Autodesk Inventor part; units mm, degrees
ref_plane "YZ Plane" through (0, 0, 0) normal (1, 0, 0) x (0, 1, 0)
ref_plane "XZ Plane" through (0, 0, 0) normal (0, 1, 0) x (-1, 0, 0)
ref_plane "XY Plane" through (0, 0, 0) normal (0, 0, 1) x (1, 0, 0)
sketch "Sketch1" plane through (0, 0, 0) normal (0, 0, 1) x (1, 0, 0)
  line L0 (-27, -64) -> (27, -64)
  line L1 (27, -64) -> (27, 64)
  line L2 (27, 64) -> (-27, 64)
  line L3 (-27, 64) -> (-27, -64)
  line L4 (-27, -64) -> (27, 64) construction
  line L5 (27, -64) -> (-27, 64) construction
  line L6 (-13, 56) -> (13, 56)
  line L7 (19, 50) -> (19, 41)
  line L8 (13, 35) -> (13, 35)
  line L9 (-19, 41) -> (-19, 50)
  arc A0 (-13, 56) -> (-19, 50) centre (-13, 50) ccw
  arc A1 (19, 50) -> (13, 56) centre (13, 50) ccw
  arc A2 (13, 35) -> (19, 41) centre (13, 41) ccw
  arc A3 (-19, 41) -> (-13, 35) centre (-13, 41) ccw
  line L10 (-37.8, 0) -> (37.8, 0) construction
  line L11 (-27, 64) -> (27, -64) construction
  line L12 (-13, -56) -> (13, -56)
  line L13 (19, -50) -> (19, -41)
  line L14 (13, -35) -> (13, -35)
  line L15 (-19, -41) -> (-19, -50)
  arc A4 (-19, -50) -> (-13, -56) centre (-13, -50) ccw
  arc A5 (13, -56) -> (19, -50) centre (13, -50) ccw
  arc A6 (19, -41) -> (13, -35) centre (13, -41) ccw
  arc A7 (-13, -35) -> (-19, -41) centre (-13, -41) ccw
  line L16 (-13, 35) -> (-13, -35)
  line L17 (13, 35) -> (13, -35)
  line L18 (0, -89.6) -> (0, 89.6) construction
  line L19 (-13, 35) -> (-13, 35)
  line L20 (13, 35) -> (-13, 35) construction
  line L21 (-13, -35) -> (-13, -35)
  line L22 (13, -35) -> (-13, -35) construction
  point P0 (0, 0)
  point P1 (0, 56)
  point P2 (0, 0)
  point P3 (13, 35)
  point P4 (13, -35)
  point P5 (-13, -35)
  point P6 (-13, 35)
  dimension "d0" = 54
  dimension "d1" = 128
  dimension "d2" = 38
  dimension "d3" = 6
  dimension "d4" = 35
  dimension "d5" = 8
  dimension "d6" = 26
extrude "Extrusion1" add sketch "Sketch1" along normal mid plane 40
fillet "Fillet1" radius 14 4 edges at (27, -64, 0) (-27, -64, 0) (-27, 64, 0) (27, 64, 0)
sketch "Sketch2" plane through (27, -50, 20) normal (1, 0, 0) x (0, 0, -1)
  line L0 (0, 0) -> (0, 100)
  line L1 (40, 100) -> (40, 0)
  arc A0 (0, 35) -> (4.6393, 30.2757) centre (20, 50) ccw
  arc A1 (0, 65) -> (0, 35) centre (20, 50) ccw construction
  arc A2 (40, 65) -> (35.3607, 69.7243) centre (20, 50) ccw
  arc A3 (40, 35) -> (40, 65) centre (20, 50) ccw construction
  line L2 (0, 65) -> (0, 35)
  line L3 (0, 15) -> (0, 85)
  line L4 (40, 85) -> (40, 15)
  line L5 (40, 65) -> (40, 35)
  circle A4 centre (20, 50) radius 18 construction
  line L6 (11.1075, 74.432) -> (20, 50) construction
  line L7 (28.8925, 74.432) -> (20, 50) construction
  line L8 (20, -39.6) -> (20, 139.6) construction
  line L9 (11.1075, 74.432) -> (28.8925, 74.432) construction
  arc A5 (26.1564, 66.9145) -> (13.8436, 66.9145) centre (20, 50) ccw
  arc A6 (4.6393, 69.7243) -> (13.8436, 66.9145) centre (11.1075, 74.432) ccw
  arc A7 (19.1075, 74.432) -> (19.0885, 74.9834) centre (11.1075, 74.432) ccw construction
  arc A8 (20.9115, 74.9834) -> (20.8925, 74.432) centre (28.8925, 74.432) ccw construction
  arc A9 (26.1564, 66.9145) -> (35.3607, 69.7243) centre (28.8925, 74.432) ccw
  arc A10 (4.6393, 69.7243) -> (0, 65) centre (20, 50) ccw
  arc A11 (35.3607, 69.7243) -> (4.6393, 69.7243) centre (20, 50) ccw construction
  line L10 (55, 50) -> (-15, 50) construction
  circle A12 centre (20, 50) radius 18 construction
  line L11 (11.1075, 25.568) -> (20, 50) construction
  line L12 (28.8925, 25.568) -> (20, 50) construction
  line L13 (20, 139.6) -> (20, -39.6) construction
  arc A13 (13.8436, 33.0855) -> (26.1564, 33.0855) centre (20, 50) ccw
  arc A14 (13.8436, 33.0855) -> (4.6393, 30.2757) centre (11.1075, 25.568) ccw
  arc A15 (35.3607, 30.2757) -> (26.1564, 33.0855) centre (28.8925, 25.568) ccw
  arc A16 (4.6393, 30.2757) -> (35.3607, 30.2757) centre (20, 50) ccw construction
  arc A17 (35.3607, 30.2757) -> (40, 35) centre (20, 50) ccw
  point P0 (20, 74.432)
  dimension "d10" = 50
  dimension "d11" = 36
  dimension "d15" = 40
extrude "Extrusion2" add sketch "Sketch2" along normal blind 12
sketch "Sketch3" plane through (39, -50, 20) normal (1, 0, 0) x (0, 0, -1)
  arc A0 (40, 65) -> (35.3607, 69.7243) centre (20, 50) ccw
  circle A1 centre (20, 50) radius 15
  dimension "d18" = 30
extrude "Extrusion3" add sketch "Sketch3" along normal blind 25
chamfer "Chamfer1" distance 2 angle 45 1 edges at (64, 0, 15)
mirror "Mirror1" about plane through (0, 0, 0) normal (1, 0, 0) of "Extrusion2", "Extrusion3", "Chamfer1"
sketch "Sketch4" plane through (-64, 0, 0) normal (-1, 0, 0) x (0, 0, 1)
  circle A0 centre (0, 0) radius 13
  point P0 (0, 0)
hole "Hole1" at (-64, 0, 0) direction (1, 0, 0) diameter 15 end through all
properties part number "Part036.Connecting cross" material "Steel, Carbon"
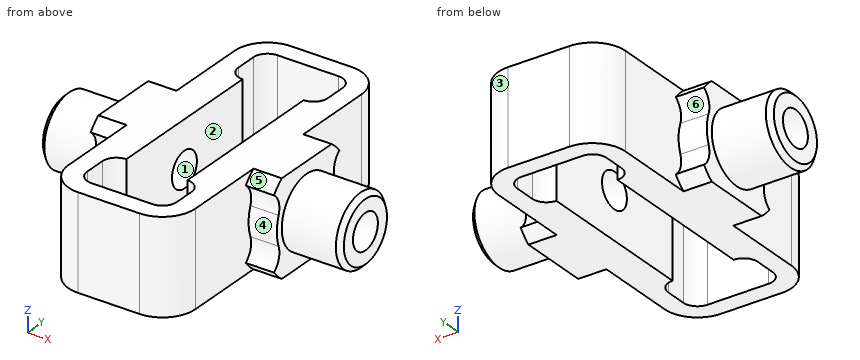
Input: part model. Units: mm. Frame: model coordinates. Face numbers are marked on the shaded views. A direction names the side the tool comes from. Give positions to 0.01 mm unless a question says otherwise; leave off trailing zeros. Order: outer loops, then holes, each group sorted by start corner. A loop starts at its lowest first (then second) coordinate and runs counter-clockwise, first axis right, second up. Notation, with made-up numbers: (67.5, -33.5) - (95.5, -33.5) arc R11 ccw to (95.5, -20.5) - close; hole circle Ø6 at (69.25, 37.25). An arc over 180 degrees is marked (long way). One line per item, written item: value.
1. Draft query along X for the marked faces 1, 2 and 3. Return one class per face: released by +X, released by -X, zero draft, split by the parting line, or undercut.
Determined:
face 1: zero draft
face 2: undercut
face 3: released by +X
2. Reachability of the marked faces 4, 5 and 6 from +Z, -Z, +X, -X, +Y, -Y: full face, straight path, thin tool, end or side. Return the list, or none.
Determined:
face 4: +X, -Y
face 5: +Z, +X, -Y
face 6: -X, +Y
3. Cut plane D-D, the plane x = -30.5. Output: boundary loops of the cut face in (y, z), and give its area (3 significant figures).
Determined:
outline: (-19.72, -15.36) arc R25 ccw to (-15, -20) - (15, -20) arc R25 ccw to (19.72, -15.36) arc R8 cw to (16.91, -6.16) arc R18 ccw to (16.91, 6.16) arc R8 cw to (19.72, 15.36) arc R25 ccw to (15, 20) - (-15, 20) arc R25 ccw to (-19.72, 15.36) arc R8 cw to (-16.91, 6.16) arc R18 ccw to (-16.91, -6.16) arc R8 cw to start; hole circle Ø15 at (0, 0)
area: 1,220 mm2
4. Line query: probe 1 along X at (y, z) = (-22, 4); probe 2 along X at (y, z) = (46.5, -14); probe 3 along Y at (x, z) = (5.5, -10). Output: solid intervals per line, ascending.
Determined:
probe 1: -27 to -13, 13 to 27
probe 2: -27 to -19, 19 to 27
probe 3: -64 to -56, 56 to 64
5. Cut plane B-B, the plane y = 0. Output: boundary loops of the cut face in (x, z), and give its area (3 significant figures).
Determined:
outline: (-64, -13) - (-62, -15) - (-39, -15) - (-39, -20) - (-13, -20) - (-13, -7.5) - (-64, -7.5) - close; (-64, 7.5) - (-13, 7.5) - (-13, 20) - (-39, 20) - (-39, 15) - (-62, 15) - (-64, 13) - close; (13, -20) - (39, -20) - (39, -15) - (62, -15) - (64, -13) - (64, -7.5) - (13, -7.5) - close; (13, 7.5) - (64, 7.5) - (64, 13) - (62, 15) - (39, 15) - (39, 20) - (13, 20) - close
area: 2,040 mm2
6. Cut plane C-C, the plane y = 25. Output: boundary loops of the cut face in (x, z).
Determined:
outline: (-27, -20) - (-13, -20) - (-13, 20) - (-27, 20) - close; (13, -20) - (27, -20) - (27, 20) - (13, 20) - close
7. Cut plane A-A, the plane x = -4.5. Output: boundary loops of the cut face in (y, z).
Determined:
outline: (-64, -20) - (-56, -20) - (-56, 20) - (-64, 20) - close; (56, -20) - (64, -20) - (64, 20) - (56, 20) - close
8. Pin query (flat end, axial travel): pin 1 Ø2 at (y, z) = (24.5, -5) entering from -X; pin 2 Ø10.5 at (y, z) = (-30, -0.5) entering from +X; pin 3 Ø12 at (x, y) = (13, 37.5) entering from -Z; pin 4 Ø17.5 at (y, z) = (-24.5, -6) entering from -X. Return the tip coordinate at first contact, or that it passes through.
Determined:
pin 1: x = -27
pin 2: x = 27
pin 3: z = -20
pin 4: x = -39
